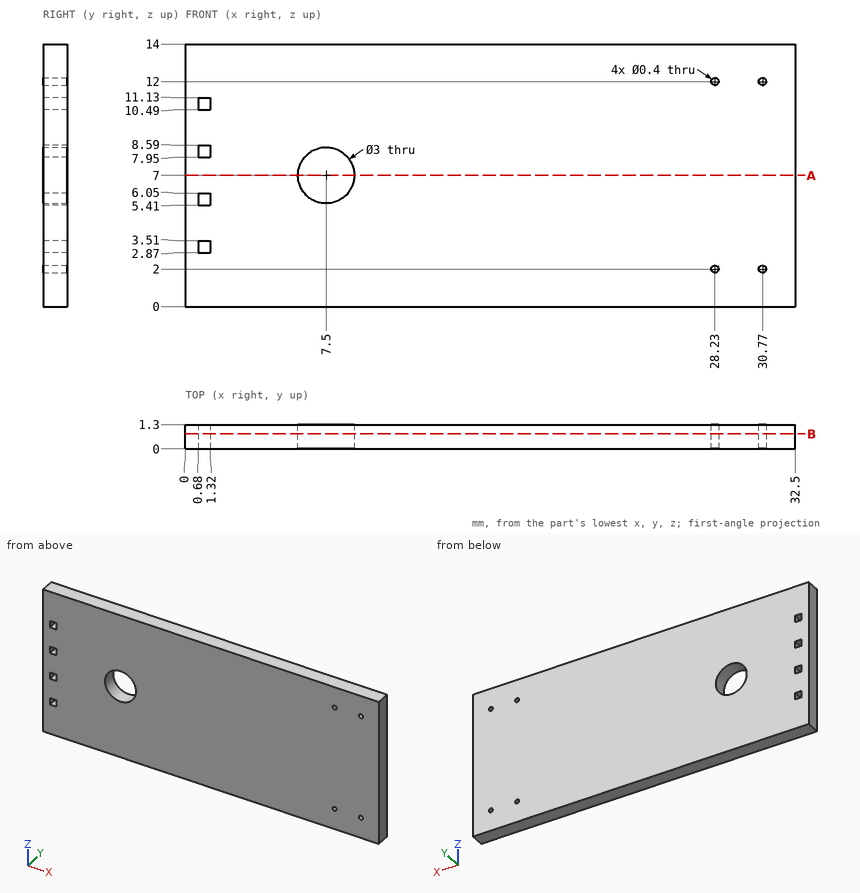
Part print with two shaded views. Sizes in mm from the minimum x, y, z corner. Coordinates: 2 decimals unless noted, no trailing zeros. Order: outer loops, then holes, each group sorted by start corner. A loop starts at its lowest first (then second) coordinate and runs counter-clockwise, first axis right, second up. Notation, with made-up numbers: (29.5, 38.25) - (57.5, 38.25) arc R20 cw to (57.5, 72.25) - close; hole circle Ø5 at (-18, 75). An arc over 180 degrees is marked (long way). Answer in a Markdown table with one row per item.
1. Drill centre lines: L1, parallel to Z at x = 30.77, y = 0.65; L2, parallel to X at y = 0.85, z = 12; L3, parallel to X at y = 0.85, z = 7. Where is each one in solid material? Low to high. Write a range as from..to.
Answer:
| item | result |
|---|---|
| L1 | 0..1.8, 2.2..11.8, 12.2..14 |
| L2 | 0..28.03, 28.43..30.57, 30.97..32.5 |
| L3 | 0..6, 9..32.5 |
2. Flat gauge pin, fed straight in: P1, Ø0.5, axis at x = 1, y = 0.5, coming from the -Z side. Where does the tip first touch, or does it go through?
Answer:
| item | result |
|---|---|
| P1 | z = 0 |
3. Slice it at B-B, the plane y = 0.8. Give the number of separate pieces and of enclosed holes in the cut face, then the cut area to 3 significant figures.
Answer:
| item | result |
|---|---|
| separate pieces | 1 |
| enclosed holes | 9 |
| area | 446 mm² |
4. Slice it at A-A, the plane z = 7. List the corners of the cut face in (x, y).
Answer:
| item | result |
|---|---|
| outline | (0, 0) - (6, 0) - (6, 1.3) - (0, 1.3) - close; (9, 0) - (32.5, 0) - (32.5, 1.3) - (9, 1.3) - close |
